from build123d import *

# Parameters (mm, degrees)
SKETCH_1_W          = 120
SKETCH_1_H          = 50
EXTRUDE_1_DEPTH     = 2
SKETCH_2_R          = 1.5
CUT_EXTRUDE_1_DEPTH = 66.030761952
FILLET_1_R          = 3
SKETCH_3_R          = 1.5
CUT_EXTRUDE_2_DEPTH = 66.030761952


with BuildPart() as part:
    # 草图1 → 凸台-拉伸1 (new body)
    with BuildSketch(Plane(origin=(0, 0, 0), x_dir=(1, 0, 0), z_dir=(0, 1, 0))):
        Rectangle(SKETCH_1_W, SKETCH_1_H)
    extrude(amount=EXTRUDE_1_DEPTH)

    # 草图2 → 切除-拉伸1 (cut, through all)
    with BuildSketch(Plane(origin=(0, 2, 0), x_dir=(1, 0, 0), z_dir=(0, 1, 0))):
        with Locations(Location((-30, 20, 0), (0, 0, 270))):
            Circle(SKETCH_2_R)
        with Locations(Location((-55, 0, 0), (0, 0, 270))):
            Circle(SKETCH_2_R)
        with Locations(Location((-30, -20, 0), (0, 0, 90))):
            Circle(SKETCH_2_R)
        with Locations(Location((30, -20, 0), (0, 0, 270))):
            Circle(SKETCH_2_R)
        with Locations(Location((55, 0, 0), (0, 0, 90))):
            Circle(SKETCH_2_R)
        with Locations(Location((30, 20, 0), (0, 0, 90))):
            Circle(SKETCH_2_R)
        with Locations(Location((-57, 22, 0), (0, 0, 270))):
            Circle(SKETCH_2_R)
        with Locations(Location((-57, -22, 0), (0, 0, 90))):
            Circle(SKETCH_2_R)
        with Locations(Location((57, -22, 0), (0, 0, 270))):
            Circle(SKETCH_2_R)
        with Locations(Location((57, 22, 0), (0, 0, 90))):
            Circle(SKETCH_2_R)
    extrude(amount=-CUT_EXTRUDE_1_DEPTH, mode=Mode.SUBTRACT)

    # 圆角1
    fillet_1_edges = [part.edges().sort_by_distance(p)[0] for p in [
        (60, 1, 25),
        (-60, 1, 25),
        (-60, 1, -25),
        (60, 1, -25),
    ]]
    fillet(fillet_1_edges, radius=FILLET_1_R)

    # 草图3 → 切除-拉伸2 (cut, through all)
    with BuildSketch(Plane(origin=(0, 2, 0), x_dir=(1, 0, 0), z_dir=(0, 1, 0))):
        with Locations((-55, 20)):
            Circle(SKETCH_3_R)
        with Locations(Location((-45, 20, 0), (0, 0, 270))):
            Circle(SKETCH_3_R)
        with Locations(Location((-35, 20, 0), (0, 0, 270))):
            Circle(SKETCH_3_R)
        with Locations(Location((-25, 20, 0), (0, 0, 270))):
            Circle(SKETCH_3_R)
        with Locations(Location((-15, 20, 0), (0, 0, 270))):
            Circle(SKETCH_3_R)
        with Locations(Location((-5, 20, 0), (0, 0, 270))):
            Circle(SKETCH_3_R)
        with Locations(Location((5, 20, 0), (0, 0, 270))):
            Circle(SKETCH_3_R)
        with Locations(Location((15, 20, 0), (0, 0, 270))):
            Circle(SKETCH_3_R)
        with Locations(Location((25, 20, 0), (0, 0, 270))):
            Circle(SKETCH_3_R)
        with Locations(Location((35, 20, 0), (0, 0, 270))):
            Circle(SKETCH_3_R)
        with Locations(Location((45, 20, 0), (0, 0, 270))):
            Circle(SKETCH_3_R)
        with Locations((55, 20)):
            Circle(SKETCH_3_R)
        with Locations(Location((-45, 10, 0), (0, 0, 270))):
            Circle(SKETCH_3_R)
        with Locations(Location((-35, 10, 0), (0, 0, 270))):
            Circle(SKETCH_3_R)
        with Locations(Location((-25, 10, 0), (0, 0, 270))):
            Circle(SKETCH_3_R)
        with Locations(Location((-15, 10, 0), (0, 0, 270))):
            Circle(SKETCH_3_R)
        with Locations(Location((-5, 10, 0), (0, 0, 270))):
            Circle(SKETCH_3_R)
        with Locations(Location((5, 10, 0), (0, 0, 270))):
            Circle(SKETCH_3_R)
        with Locations(Location((15, 10, 0), (0, 0, 270))):
            Circle(SKETCH_3_R)
        with Locations(Location((25, 10, 0), (0, 0, 270))):
            Circle(SKETCH_3_R)
        with Locations(Location((35, 10, 0), (0, 0, 270))):
            Circle(SKETCH_3_R)
        with Locations(Location((45, 10, 0), (0, 0, 270))):
            Circle(SKETCH_3_R)
        with Locations(Location((55, 10, 0), (0, 0, 270))):
            Circle(SKETCH_3_R)
        with Locations(Location((-45, 0, 0), (0, 0, 270))):
            Circle(SKETCH_3_R)
        with Locations(Location((-35, 0, 0), (0, 0, 270))):
            Circle(SKETCH_3_R)
        with Locations(Location((-25, 0, 0), (0, 0, 270))):
            Circle(SKETCH_3_R)
        with Locations(Location((-15, 0, 0), (0, 0, 270))):
            Circle(SKETCH_3_R)
        with Locations(Location((-5, 0, 0), (0, 0, 270))):
            Circle(SKETCH_3_R)
        with Locations(Location((5, 0, 0), (0, 0, 270))):
            Circle(SKETCH_3_R)
        with Locations(Location((15, 0, 0), (0, 0, 270))):
            Circle(SKETCH_3_R)
        with Locations(Location((25, 0, 0), (0, 0, 270))):
            Circle(SKETCH_3_R)
        with Locations(Location((35, 0, 0), (0, 0, 270))):
            Circle(SKETCH_3_R)
        with Locations(Location((45, 0, 0), (0, 0, 270))):
            Circle(SKETCH_3_R)
        with Locations(Location((55, 0, 0), (0, 0, 90))):
            Circle(SKETCH_3_R)
        with Locations(Location((-45, -10, 0), (0, 0, 270))):
            Circle(SKETCH_3_R)
        with Locations(Location((-35, -10, 0), (0, 0, 270))):
            Circle(SKETCH_3_R)
        with Locations(Location((-25, -10, 0), (0, 0, 270))):
            Circle(SKETCH_3_R)
        with Locations(Location((-15, -10, 0), (0, 0, 270))):
            Circle(SKETCH_3_R)
        with Locations(Location((-5, -10, 0), (0, 0, 270))):
            Circle(SKETCH_3_R)
        with Locations(Location((5, -10, 0), (0, 0, 270))):
            Circle(SKETCH_3_R)
        with Locations(Location((15, -10, 0), (0, 0, 270))):
            Circle(SKETCH_3_R)
        with Locations(Location((25, -10, 0), (0, 0, 270))):
            Circle(SKETCH_3_R)
        with Locations(Location((35, -10, 0), (0, 0, 270))):
            Circle(SKETCH_3_R)
        with Locations(Location((45, -10, 0), (0, 0, 270))):
            Circle(SKETCH_3_R)
        with Locations(Location((55, -10, 0), (0, 0, 270))):
            Circle(SKETCH_3_R)
        with Locations(Location((-45, -20, 0), (0, 0, 270))):
            Circle(SKETCH_3_R)
        with Locations(Location((-35, -20, 0), (0, 0, 270))):
            Circle(SKETCH_3_R)
        with Locations(Location((-25, -20, 0), (0, 0, 270))):
            Circle(SKETCH_3_R)
        with Locations(Location((-15, -20, 0), (0, 0, 270))):
            Circle(SKETCH_3_R)
        with Locations(Location((-5, -20, 0), (0, 0, 270))):
            Circle(SKETCH_3_R)
        with Locations(Location((5, -20, 0), (0, 0, 270))):
            Circle(SKETCH_3_R)
        with Locations(Location((15, -20, 0), (0, 0, 270))):
            Circle(SKETCH_3_R)
        with Locations(Location((25, -20, 0), (0, 0, 270))):
            Circle(SKETCH_3_R)
        with Locations(Location((35, -20, 0), (0, 0, 270))):
            Circle(SKETCH_3_R)
        with Locations(Location((45, -20, 0), (0, 0, 270))):
            Circle(SKETCH_3_R)
        with Locations((55, -20)):
            Circle(SKETCH_3_R)
        with Locations(Location((-55, 10, 0), (0, 0, 270))):
            Circle(SKETCH_3_R)
        with Locations(Location((-55, 0, 0), (0, 0, 270))):
            Circle(SKETCH_3_R)
        with Locations(Location((-55, -10, 0), (0, 0, 270))):
            Circle(SKETCH_3_R)
        with Locations((-55, -20)):
            Circle(SKETCH_3_R)
    extrude(amount=-CUT_EXTRUDE_2_DEPTH, mode=Mode.SUBTRACT)


solid = part.part
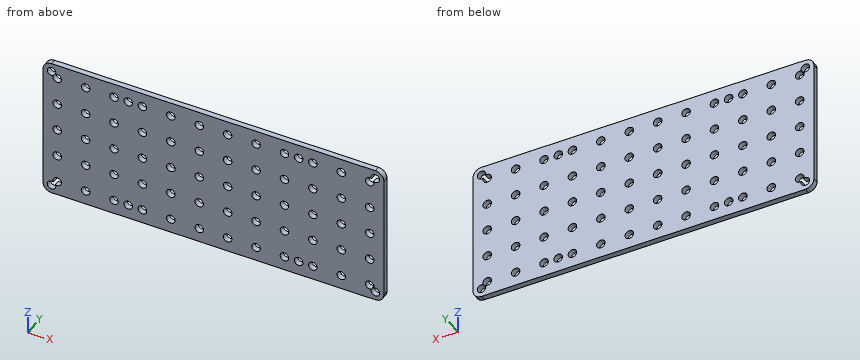
For this review, take the finished solid that the model builds, in its own axes (mm). Round coordinates to 2 decimals unless told otherwise and drop trailing zeros. Order: outer loops, then holes, each group sorted by start corner. A loop starts at its lowest first (then second) coordinate and runs counter-clockwise, first axis right, second up. Notation, with made-up numbers: (59.5, -12.5) -> (114.5, -12.5) arc R23 ccw to (114.5, 17.5) -> close; hole circle Ø7 at (16.5, 71.5). An arc over 180 degrees is marked (long way). Put each result on its own line as item: value.
Q1. Add section C-C on z = 10. State how many separate pieces and enclosed holes the cut face has, plus the area to 3 significant figures.
Check result:
separate pieces: 13
enclosed holes: 0
area: 168 mm2
Q2. For probe 1 along Z at (x, y) = (-14.5, 1), list the stretches that pass through material, from the lowest coordinate up. Write a range as [from, to].
Check result:
probe 1: [-25, -21.41], [-18.59, -11.41], [-8.59, -1.41], [1.41, 8.59], [11.41, 18.59], [21.41, 25]
Q3. Insertion check: pin 1 Ø2.5 at (x, z) = (45, 0) entering from -Y. The pin has a flat end and moves straight along its axis. Give the tip position at first contact, or say it passes through.
Check result:
pin 1: through
Q4. Add section B-B on x = -30. Write out the cut boundary in (y, z).
Check result:
outline: (0, -25) -> (2, -25) -> (2, -21.5) -> (0, -21.5) -> close; (0, -18.5) -> (2, -18.5) -> (2, 18.5) -> (0, 18.5) -> close; (0, 21.5) -> (2, 21.5) -> (2, 25) -> (0, 25) -> close
Q5. Add section A-A on x = 5. Write out the cut boundary in (y, z).
Check result:
outline: (0, -25) -> (2, -25) -> (2, -21.5) -> (0, -21.5) -> close; (0, -18.5) -> (2, -18.5) -> (2, -11.5) -> (0, -11.5) -> close; (0, -8.5) -> (2, -8.5) -> (2, -1.5) -> (0, -1.5) -> close; (0, 1.5) -> (2, 1.5) -> (2, 8.5) -> (0, 8.5) -> close; (0, 11.5) -> (2, 11.5) -> (2, 18.5) -> (0, 18.5) -> close; (0, 21.5) -> (2, 21.5) -> (2, 25) -> (0, 25) -> close
